Check sheet for the modelled part. Datum: model origin and axes. Units: mm. Face numbers are marked on the shaded views. Give positions to 0.01 mm unless a question says otherwise; leave off trailing zeros. Loops run counter-clockwise (first coordinate to the right, second up) from the corner with the lowest first, then second, coordinate; pieces in that order, holes last. Notation, with made-up numbers: M 72.5,-14 L 111.5,-14 A25 ccw 111.5,1 Z; hole C 18,42.25 d1. An arc over 180 degrees is marked long. Write each question's results on one line, items separated by ' | '. Start each with the question number.
1. Draft check along Z on the marked faces 1 and 2. Enter one of: pulls with the +Z half, pulls with the -Z half, needs draft (parallel to the pull), parting line crosses it, or undercut.
2. Sectioned sample at D-D on z = 12. Record the cut outline in (x, y), and give its area (3 significant figures).
3. Go/stop test with flat-tipped pins: pin 1 (2 mm diameter, centred on x = -6, z = -10, fed in from +Y); pin 2 (10.5 mm diameter, centred on x = 0, z = -3, fed in from -Y). Record where each tip stops, or that it passes through.
4. Sectioned sample at A-A on z = 0. Record the cut outline in (x, y), and give its area (3 significant figures).
5. Sectioned sample at B-B on x = 0. Record the cut outline in (y, z).
6. Material ranges on line 1 along Z through (x, y) = (0, 0.25); line 2 along Z through (x, y) = (0, 1.3), recorded low to high.
7. Sectioned sample at C-C on y = 0.75. Record the cut outline in (x, z).
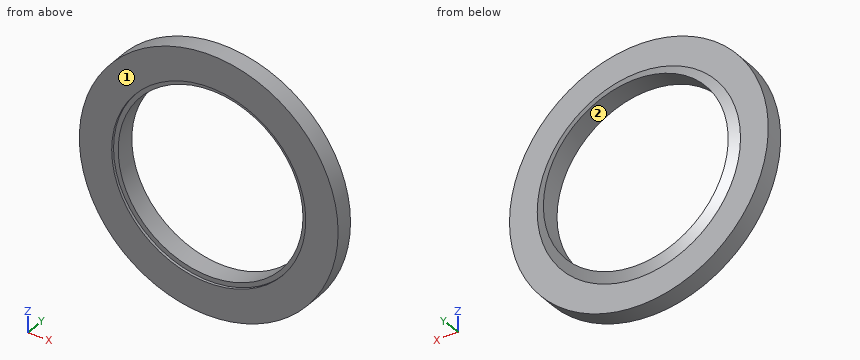
```python
from build123d import *

# Parameters (mm, degrees)
SKETCH2_R          = 10.5
SKETCH2_R_2        = 10
CUT_EXTRUDE1_DEPTH = 0.3


with BuildPart() as part:
    # Sketch1 → Revolve1 (revolve)
    with BuildSketch(Plane.XY):
        Polygon((10, 0), (14, 0), (14, 2), (11, 2), (10, 2), align=None)
        Polygon((10, 2), (11, 2), (10, 2.5), align=None)
    revolve(axis=Axis((0, 0, 0), (0, 1, 0)))

    # Sketch2 → Cut-Extrude1 (cut)
    with BuildSketch(Plane.XZ):
        Circle(SKETCH2_R)
        Circle(SKETCH2_R_2, mode=Mode.SUBTRACT)
    extrude(amount=-CUT_EXTRUDE1_DEPTH, mode=Mode.SUBTRACT)


solid = part.part
```
Output values:
1) face 1: needs draft | face 2: undercut
2) outline: M -7.21,0 L 7.21,0 L 7.21,2 L -7.21,2 Z | area: 28.8 mm2
3) pin 1: y = 2.17 | pin 2: through
4) outline: M -14,0 L -10.5,0 L -10.5,0.3 L -10,0.3 L -10,2.5 L -11,2 L -14,2 Z; M 10,0.3 L 10.5,0.3 L 10.5,0 L 14,0 L 14,2 L 11,2 L 10,2.5 Z | area: 16.2 mm2
5) outline: M 0,-14 L 2,-14 L 2,-11 L 2.5,-10 L 0.3,-10 L 0.3,-10.5 L 0,-10.5 Z; M 0,10.5 L 0.3,10.5 L 0.3,10 L 2.5,10 L 2,11 L 2,14 L 0,14 Z
6) line 1: -14 to -10.5, 10.5 to 14 | line 2: -14 to -10, 10 to 14
7) outline: C 0,0 d28; hole C 0,0 d20
